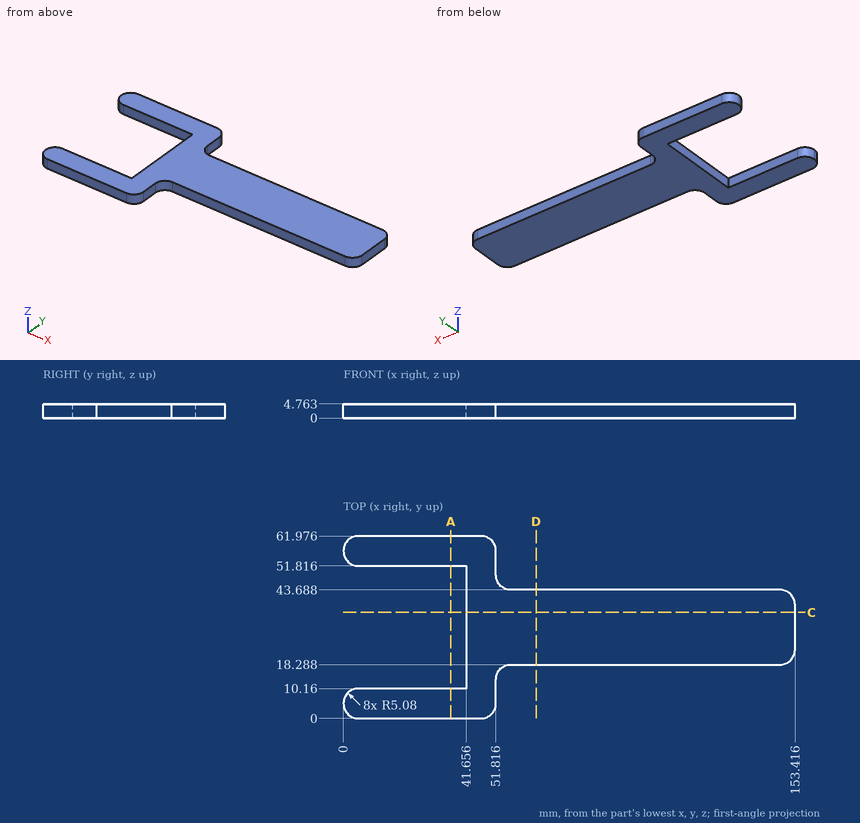
Can you work these out from the drawing? Everything is in mm from the part's minimum corner. Coordinates: 2 decimals unless noted, no trailing zeros. Loops run counter-clockwise (first coordinate to the right, second up) from the corner with the lowest first, then second, coordinate; pieces in that order, holes last.
1. I need wall thicknesses on L1, parallel to Y at x = 9.5, z = 1.6 (1 decimal); L2, parallel to X at y = 37.5, z = 4.2 (1 decimal); L3, parallel to Y at x = 98, z = 3.1. Which ranges of each line are inside material? Lowest first, please.
2. Imagine slicing it at C-C, the plane y = 36. Please give me the cut outline in (x, z) (1 decimal).
3. Imagine slicing it at D-D, the plane x = 65.5. Please give me the cut outline in (y, z), and give its area (3 significant figures).
4. Imagine slicing it at A-A, the plane x = 36.5. Please give me the cut outline in (y, z) (1 decimal).
5. For P1, Ø1.5, axis at y = 18, z = 4, coming from the -X side; P2, Ø1.4, axis at x = 125.5, z = 2, coming from the -Y side; P3, Ø2.5, axis at x = 28.5, z = 2, coming from the -Y side; P4, Ø1.4, axis at x = 123, z = 2, coming from the +Y side, each with a flat end and sliding along its axis, tell me the tip position at first contact or that it passes through.
Taken from the geometry:
1. L1: y = 0 to 10.2, 51.8 to 62
1. L2: x = 41.7 to 153.4
1. L3: y = 18.29 to 43.69
2. outline: (41.7, 0) - (153.4, 0) - (153.4, 4.8) - (41.7, 4.8) - close
3. outline: (18.29, 0) - (43.69, 0) - (43.69, 4.76) - (18.29, 4.76) - close
3. area: 121 mm2
4. outline: (0, 0) - (10.2, 0) - (10.2, 4.8) - (0, 4.8) - close; (51.8, 0) - (62, 0) - (62, 4.8) - (51.8, 4.8) - close
5. P1: stops at x = 41.66
5. P2: stops at y = 18.29
5. P3: stops at y = 0
5. P4: stops at y = 43.69
